The listing builds one solid part. Answer for the finished solid, in the listing's coordinates (mm). Face numbers are marked on the shaded views. A direction names the side the tool comes from. Give positions to 0.01 mm unless a question says otherwise; leave off trailing zeros. Write each loop counter-clockwise with the first axis right and the second up, starting at its lowest first coordinate (ties: lowest second). Pieces come first, ordered by that corner, then holes. Notation, with made-up numbers: (52.25, 76) - (60.25, 76) arc R27 cw to (60.25, 109) - close; hole circle Ø8 at (-1.5, 6). An arc over 180 degrees is marked (long way). Answer in a Markdown table with one row per item. Add a question column.
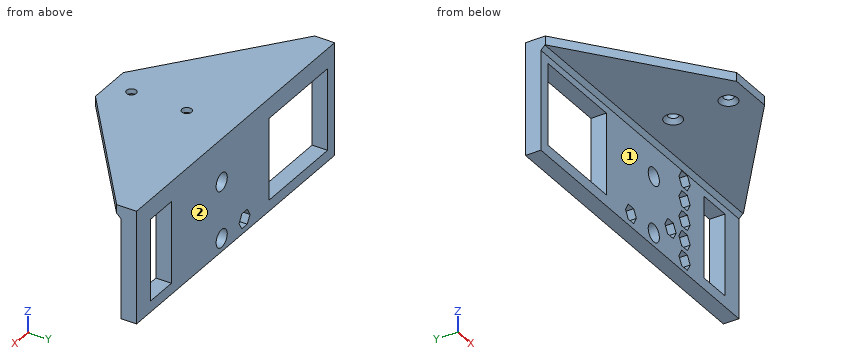
from build123d import *

# Parameters (mm, degrees)
SKETCH_W            = 142.082904
SKETCH_H            = 47
SKETCH_R            = 4
SKETCH_W_2          = 42
SKETCH_H_2          = 37
SKETCH_W_3          = 15
PAD_DEPTH           = 7
POCKET_DEPTH        = 6.5
LINEARPATTERN_COUNT = 5
LINEARPATTERN_PITCH = 9
POCKET001_DEPTH     = 6.5
PAD001_DEPTH        = 4
CHAMFER_SIZE        = 1.8
HOLE_D              = 4.4
HOLE_DEPTH          = 25
HOLE_CSINK_D        = 8
HOLE_CSINK_ANGLE    = 90
POCKET002_DEPTH     = 7.001


with BuildPart() as part:
    # Sketch → Pad (new body)
    with BuildSketch(Plane.XZ):
        with Locations((71.041452, 23.5)):
            Rectangle(SKETCH_W, SKETCH_H)
        with Locations((81, 31.5)):
            Circle(SKETCH_R, mode=Mode.SUBTRACT)
        with Locations((81, 6)):
            Circle(SKETCH_R, mode=Mode.SUBTRACT)
        with Locations((26, 23.5)):
            Rectangle(SKETCH_W_2, SKETCH_H_2, mode=Mode.SUBTRACT)
        with Locations((124.582904, 23.5)):
            Rectangle(SKETCH_W_3, SKETCH_H_2, mode=Mode.SUBTRACT)
    extrude(amount=PAD_DEPTH)

    # Sketch001 (on Face16 of Pad) → Pocket (cut)
    with BuildSketch(Plane.XZ.offset(7)):
        Polygon((105.062178, 45), (101.020726, 45), (99, 41.5), (101.020726, 38), (105.062178, 38), (107.082904, 41.5), align=None)
    pocket = extrude(amount=-POCKET_DEPTH, mode=Mode.SUBTRACT)

    # LinearPattern: Pocket ×5
    with Locations(*[(0, 0, -i * LINEARPATTERN_PITCH) for i in range(1, LINEARPATTERN_COUNT)]):
        add(pocket, mode=Mode.SUBTRACT)

    # Sketch002 (on Face5 of LinearPattern) → Pocket001 (cut)
    with BuildSketch(Plane.XZ.offset(7)):
        Polygon((94.979274, 11), (97, 14.5), (94.979274, 18), (90.937822, 18), (88.917096, 14.5), (90.937822, 11), align=None)
    extrude(amount=-POCKET001_DEPTH, mode=Mode.SUBTRACT)

    # Sketch003 (on Face1 of Pocket001) → Pad001 (join)
    with BuildSketch(Plane(origin=(0, 0, 47), x_dir=(-1, 0, 0), z_dir=(0, 0, 1))):
        Polygon((-142.082904, 9), (-81.041452, 57), (-61.041452, 57), (0, 9), (0, 0), (-142.082904, 0), align=None)
    extrude(amount=PAD001_DEPTH)

    # Chamfer
    chamfer_edges = [part.edges().sort_by_distance(p)[0] for p in [
        (71.041452, -7, 47),
    ]]
    chamfer(chamfer_edges, length=CHAMFER_SIZE)

    # Hole
    with Locations(Plane(origin=(0, 0, 47), x_dir=(1, 0, 0), z_dir=(0, 0, -1))):
        with Locations((71.041452, 47), (71.041452, 22)):
            CounterSinkHole(HOLE_D / 2, HOLE_CSINK_D / 2, depth=HOLE_DEPTH, counter_sink_angle=HOLE_CSINK_ANGLE)

    # Sketch005 (on Face2 of Hole) → Pocket002 (cut, through all)
    with BuildSketch(Plane.XZ.offset(7)):
        Polygon((66.55, 2.5), (68.5, 5.877499), (66.55, 9.254998), (62.65, 9.254998), (60.7, 5.877499), (62.65, 2.5), align=None)
    extrude(amount=-POCKET002_DEPTH, mode=Mode.SUBTRACT)


solid = part.part
1. Section D-D (y = -5) is taken. State how many separate pieces and enclosed holes the cut face has, and give its area (3 significant figures).
2. Straight lines are drawn through the part: L1, parallel to Z at x = 81, y = -5.5; L2, parallel to Z at x = 36, y = -4; L3, parallel to Y at x = 93.5, z = 31. For each, find the intervals that lie inside material, in ascending order. Write a range as [from, to].
3. A tool of negligible diameter and unlimited length cuts with its end or side. For the marked faces 1 and 2, from which of +Z, -Z, +X, -X, +Y, -Y can it reach the whole face along a straight path? Write none if from no direction.
4. Section A-A (z = 13) is taken. Give the vertices of the cut face in (x, y).
5. Section C-C (x = 29) is taken. Give the vertices of the cut face in (y, z), and give its area (3 significant figures).
6. Given pin 1 Ø3 at (x, y) = (104, -5) entering from -Z; pin 2 Ø4 at (x, z) = (50, 45.5) entering from -Y; pin 3 Ø8 at (x, y) = (59, -49) entering from -Z; pin 4 Ø5.5 at (x, z) = (92, 14.5) entering from -Y, each flat-ended and moving along its own axis, determine where each tip first touches the part or whether it passes through.
7. Section B-B (y = -47) is taken. Give the vertices of the cut face in (x, z).
Geometry check:
| question | item | result |
|---|---|---|
| 1 | separate pieces | 1 |
| 1 | enclosed holes | 11 |
| 1 | area | 4,740 mm² |
| 2 | L1 | [0, 2], [10, 27.5], [35.5, 51] |
| 2 | L2 | [0, 5], [42, 51] |
| 2 | L3 | [-7, 0] |
| 3 | face 1 | -Z, +X, -X, -Y |
| 3 | face 2 | +Z, -Z, +X, -X, +Y |
| 4 | outline | (0, -7) - (5, -7) - (5, 0) - (0, 0) - close; (47, -7) - (89.78, -7) - (89.78, -0.5) - (96.13, -0.5) - (96.13, -7) - (99.87, -7) - (99.87, -0.5) - (106.22, -0.5) - (106.22, -7) - (117.08, -7) - (117.08, 0) - (47, 0) - close; (132.08, -7) - (142.08, -7) - (142.08, 0) - (132.08, 0) - close |
| 5 | outline | (-31.8, 47) - (-8.8, 47) - (-7, 45.2) - (-7, 42) - (0, 42) - (0, 51) - (-31.8, 51) - close; (-7, 0) - (0, 0) - (0, 5) - (-7, 5) - close |
| 5 | area | 199 mm² |
| 6 | pin 1 | z = 0 |
| 6 | pin 2 | y = -49.36 |
| 6 | pin 3 | z = 47 |
| 6 | pin 4 | y = -7 |
| 7 | outline | (48.32, 47) - (67.04, 47) - (68.84, 48.8) - (68.84, 51) - (48.32, 51) - close; (73.24, 48.8) - (75.04, 47) - (93.76, 47) - (93.76, 51) - (73.24, 51) - close |
